from build123d import *

# Parameters (mm, degrees)
SKETCH3_R           = 1.5
BOSS_EXTRUDE1_DEPTH = 5
SKETCH4_R           = 1
CUT_EXTRUDE1_DEPTH  = 8.04531685
FILLET1_R           = 0.5


with BuildPart() as part:
    # Sketch2 → Revolve2 (revolve)
    with BuildSketch(Plane(origin=(0, 0, 0), x_dir=(0, 0, -1), z_dir=(1, 0, 0))):
        with BuildLine():
            Line((0, 1.54531685), (0, 0))
            Line((0, 0), (0, -0.5))
            Line((0, -0.5), (-3.730724896, -0.5))
            Line((-3.730724896, -0.5), (-3.730724896, 0))
            ThreePointArc((-3.730724896, 0), (-2.019053765, 1.143702085), (0, 1.54531685))
        make_face()
    revolve(axis=Axis((0, -0.5, 0), (0, 1, 0)))

    # Sketch3 → Boss-Extrude1 (add)
    with BuildSketch(Plane.XZ.offset(0.5)):
        Circle(SKETCH3_R)
    extrude(amount=BOSS_EXTRUDE1_DEPTH)

    # Sketch4 → Cut-Extrude1 (cut, through all)
    with BuildSketch(Plane.XZ.offset(5.5)):
        Circle(SKETCH4_R)
    extrude(amount=-CUT_EXTRUDE1_DEPTH, mode=Mode.SUBTRACT)

    # Fillet1
    fillet1_edges = [part.edges().sort_by_distance(p)[0] for p in [
        (-0.707106781, 1.449682086, -0.707106781),
    ]]
    fillet(fillet1_edges, radius=FILLET1_R)


solid = part.part
The model under review builds one solid part; all positions refer to its coordinate system, in mm. Coordinates: 2 decimals unless noted, no trailing zeros. Loops run counter-clockwise (first coordinate to the right, second up) from the corner with the lowest first, then second, coordinate; pieces in that order, holes last. Notation, with made-up numbers: M -28.5,-0.5 L 23.5,-0.5 A29 ccw 23.5,30.5 Z; hole C 63.5,82.5 d6. An arc over 180 degrees is marked long. Put each result on its own line as item: value. Start each with the question number.
Q1. Add section C-C (z = -2.75). Write out the cut boundary in (x, y), and give its area (3 significant figures).
Q2. The part is to be moulded in two halves that separate along Z. For faces 1 (the cylindrical face through (1, -2, 0)), 2 (the flat face through (0, -0.5, -2)), 3 (the cylindrical face through (-1.5, -2.96, 0.07)), say which applies: +Z half, -Z half, draft (parallel to the pull), parting line (faces both ways), or undercut.
Q3. Wall thickness on line 1 (Z direction, x = 0, y = -1); line 2 (X direction, y = -1.25, z = -0.75); line 3 (Z direction, x = 1.25, y = -0.75): over which ranges is each line inside the solid? List them lowest first.
Q4. Clearance check with a flat-ended pin moving along its axis: pin 1 (1.5 mm diameter, centred on y = -4.5, z = 0.5, fed in from +X). State where the tip first meets the part, or that it passes through.
Q5. Add section B-B (x = 2). Write out the cut boundary in (y, z), and give its area (3 significant figures).
Q6. Add section A-A (y = -1.75). Write out the cut boundary in (x, z), and give its area (3 significant figures).
Q7. Add section D-D (y = 0.5). Write out the cut boundary in (x, z).
Answers:
1. outline: M -2.52,-0.5 L 2.52,-0.5 L 2.52,0 A4.5 ccw -2.52,0 Z
1. area: 5.16 mm^2
2. face 1: undercut
2. face 2: draft
2. face 3: parting line
3. line 1: z = -1.5 to -1, 1 to 1.5
3. line 2: x = -1.3 to -0.66, 0.66 to 1.3
3. line 3: z = -0.83 to 0.83
4. pin 1: stops at x = 1.5
5. outline: M -0.5,-3.15 L 0,-3.15 A4.88 ccw 0,3.15 L -0.5,3.15 Z
5. area: 8.11 mm^2
6. outline: C 0,0 d3; hole C 0,0 d2
6. area: 3.93 mm^2
7. outline: C 0,0 d6.3; hole C 0,0 d2
